from build123d import *

# Parameters (mm, degrees)
SKETCH_1_W                  = 12
SKETCH_1_H                  = 87
EXTRUDE_1_DEPTH             = 10
HOLE_WIZARD_3_1_3_1_1_D     = 3.1
HOLE_WIZARD_3_1_3_1_1_DEPTH = 10
HOLE_WIZARD_2_7_2_7_1_D     = 2.7
HOLE_WIZARD_2_7_2_7_1_DEPTH = 12


with BuildPart() as part:
    # 草圖1 → 填料-伸長1 (new body)
    with BuildSketch(Plane(origin=(5, 0, 0), x_dir=(0, 0, -1), z_dir=(1, 0, 0))):
        with Locations((0, 43.5)):
            Rectangle(SKETCH_1_W, SKETCH_1_H)
    extrude(amount=-EXTRUDE_1_DEPTH)

    # Ø3.1 (3.1) 直徑孔1
    with Locations(Plane(origin=(5, 0, 0), x_dir=(0, 0, -1), z_dir=(1, 0, 0))):
        with Locations((1, 63.53), (1, 43.21), (1, 22.89), (1, 53.37), (1, 33.05), (1, 12.73), (1, 73.69)):
            Hole(HOLE_WIZARD_3_1_3_1_1_D / 2, depth=HOLE_WIZARD_3_1_3_1_1_DEPTH)

    # Ø2.7 (2.7) 直徑孔1
    with Locations(Plane.XY.offset(6)):
        with Locations((0, 60.1), (0, 6)):
            Hole(HOLE_WIZARD_2_7_2_7_1_D / 2, depth=HOLE_WIZARD_2_7_2_7_1_DEPTH)


solid = part.part
For this review, take the finished solid that the model builds, in its own axes (mm). Coordinates: 2 decimals unless noted, no trailing zeros. Loops run counter-clockwise (first coordinate to the right, second up) from the corner with the lowest first, then second, coordinate; pieces in that order, holes last. Notation, with made-up numbers: (74, 47.25) - (79, 47.25) arc R22 ccw to (79, 73.25) - close; hole circle Ø6 at (20.5, 80). An arc over 180 degrees is marked (long way). Use a Markdown table: item, result. Add a question column.
Item 1: We need section D-D (y = 53.37). Give the boundary of the cut face in (x, z), and give its area (3 significant figures).
Item 2: Insertion check: pin 1 Ø1.9 at (y, z) = (63.53, -1) entering from +X. The pin has a flat end and moves straight along its axis. Give the tip position at first contact, or say it passes through.
Item 3: We need section A-A (z = -1). Give the number of separate pieces and of enclosed holes in the cut face, and give its area (3 significant figures).
Item 4: We need section B-B (y = 6). Give the boundary of the cut face in (x, z), and give its area (3 significant figures).
Item 5: For line 1 (Y direction, x = -1, z = -4.5); line 2 (Z direction, x = -4.25, y = 74); line 3 (Y direction, x = -0.75, z = -4), list the stretches that pass through material, from the lowest coordinate up.
Item 6: Mouldability with a two-part tool opening along Y and no side actions: class faces 1 (the face through (0.176, 7.339, -0.084)), 2 (the face through (0, 0, 0)), 3 (the face through (0, 87, 0)), 4 (the face through (-0.07, 14.267, -1.202)) as pulls with the +Y half, pulls with the -Y half, needs draft (parallel to the pull), parting line crosses it, or undercut.
Results list:
| question | item | result |
|---|---|---|
| 1 | outline | (-5, -6) - (5, -6) - (5, -2.55) - (-5, -2.55) - close; (-5, 0.55) - (5, 0.55) - (5, 6) - (-5, 6) - close |
| 1 | area | 89.0 mm^2 |
| 2 | pin 1 | passes through |
| 3 | separate pieces | 8 |
| 3 | enclosed holes | 2 |
| 3 | area | 642 mm^2 |
| 4 | outline | (-5, -6) - (-1.35, -6) - (-1.35, 6) - (-5, 6) - close; (1.35, -6) - (5, -6) - (5, 6) - (1.35, 6) - close |
| 4 | area | 87.6 mm^2 |
| 5 | line 1 | y = 0 to 5.09, 6.91 to 59.19, 61.01 to 87 |
| 5 | line 2 | z = -6 to -2.52, 0.52 to 6 |
| 5 | line 3 | y = 0 to 4.88, 7.12 to 58.98, 61.22 to 87 |
| 6 | face 1 | undercut |
| 6 | face 2 | pulls with the -Y half |
| 6 | face 3 | pulls with the +Y half |
| 6 | face 4 | undercut |
